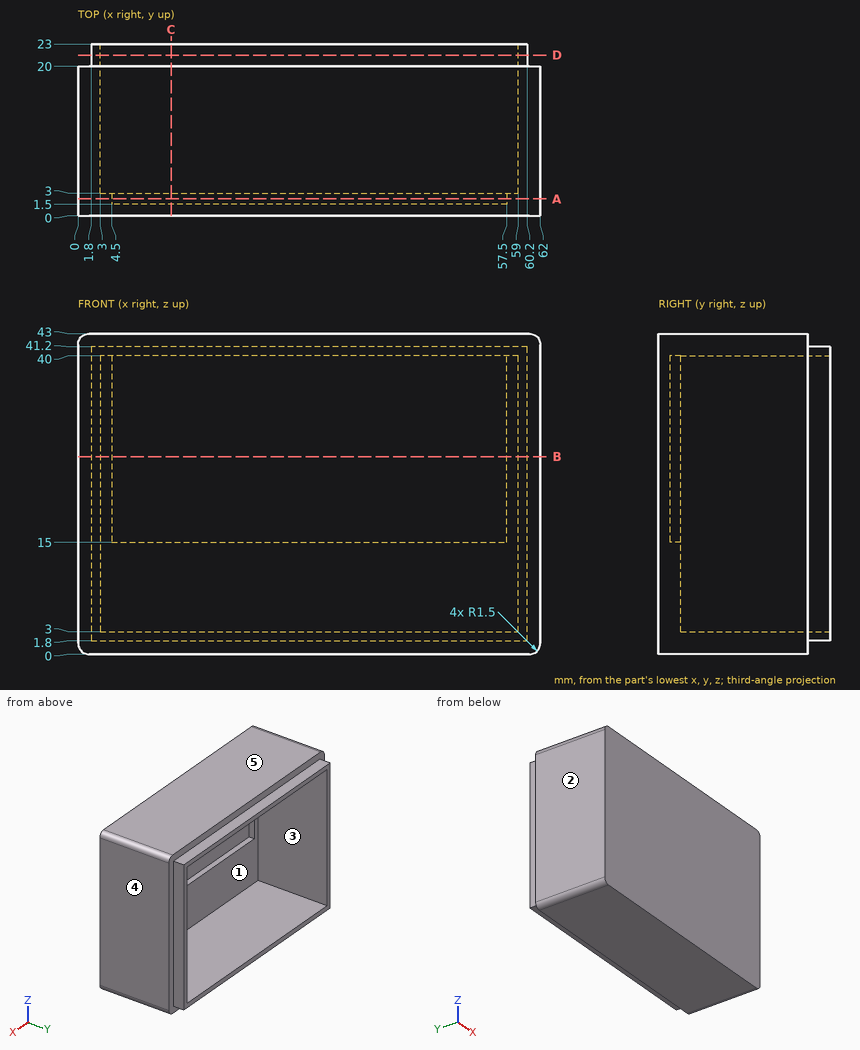
Here's the drawing with two shaded views (mm, measured from the low corner). I have some questions. A direction names the side the tool comes from. Give positions to 0.01 mm unless a question says otherwise; leave off trailing zeros. Loops run counter-clockwise (first coordinate to the right, second up) from the corner with the lowest first, then second, coordinate; pieces in that order, holes last. Notation, with made-up numbers: (-16.75, 74.5) - (19.25, 74.5) arc R19 ccw to (19.25, 83.5) - close; hole circle Ø3 at (50.25, 56.5). An arc over 180 degrees is marked (long way). One line per item, written item: value.
(1) If we section it at D-D, the plane y = 21.5: List the corners of the cut face in (x, z) for me.
Verdict:
outline: (1.8, 1.8) - (60.2, 1.8) - (60.2, 41.2) - (1.8, 41.2) - close; hole (3, 3) - (59, 3) - (59, 40) - (3, 40) - close
(2) If we mould it in two halves opening along X, with no side actions, what happens to the marked faces 3, 4 and 5? For each: released by +X, released by -X, zero draft, split by the parting line, or undercut.
Verdict:
face 3: undercut
face 4: released by +X
face 5: zero draft
(3) On a 3-axis mill with a long thin cutter (end or side, diameter ignored), from which of +Z, -Z, +X, -X, +Y, -Y can I reach the whole of each face in a straight line? I mean the marked faces 1 and 2. Say none if no direction works.
Verdict:
face 1: +Y
face 2: +Z, -Z, -X, +Y, -Y
(4) I need wall thicknesses on line 1 along X through (y, z) = (15.5, 29.5); line 2 along Z through (x, y) = (46.5, 3.5); line 3 along X through (y, z) = (2.5, 23). Which ranges of each line are inside material? Lowest first, please.
Verdict:
line 1: 0 to 3, 59 to 62
line 2: 0 to 3, 40 to 43
line 3: 0 to 4.5, 57.5 to 62
(5) If we section it at B-B, the plane z = 26.5: List the corners of the cut face in (x, y) for me.
Verdict:
outline: (0, 0) - (62, 0) - (62, 20) - (60.2, 20) - (60.2, 23) - (59, 23) - (59, 3) - (57.5, 3) - (57.5, 1.5) - (4.5, 1.5) - (4.5, 3) - (3, 3) - (3, 23) - (1.8, 23) - (1.8, 20) - (0, 20) - close
(6) If we section it at A-A, the plane y = 2.25: List the corners of the cut face in (x, z) for me.
Verdict:
outline: (0, 1.5) arc R1.5 ccw to (1.5, 0) - (60.5, 0) arc R1.5 ccw to (62, 1.5) - (62, 41.5) arc R1.5 ccw to (60.5, 43) - (1.5, 43) arc R1.5 ccw to (0, 41.5) - close; hole (4.5, 15) - (57.5, 15) - (57.5, 40) - (4.5, 40) - close
(7) If we section it at C-C, the plane x = 12.5: List the corners of the cut face in (y, z) for me, plus the area to 3 significant figures.
Verdict:
outline: (0, 0) - (20, 0) - (20, 1.8) - (23, 1.8) - (23, 3) - (3, 3) - (3, 15) - (1.5, 15) - (1.5, 40) - (23, 40) - (23, 41.2) - (20, 41.2) - (20, 43) - (0, 43) - close
area: 201 mm^2
(8) I'm going to push flat-ended pins straight in: pin 1 (7.5 mm diameter, centred on x = 19, z = 28.5, fed in from +Y); pin 2 (2.5 mm diameter, centred on x = 23.5, y = 22, fed in from +Z); pin 3 (1.5 mm diameter, centred on y = 22, z = 29.5, fed in from -X). Where does each tip first touch, or does it pass through?
Verdict:
pin 1: y = 1.5
pin 2: z = 41.2
pin 3: x = 1.8
